```python
from build123d import *

# Parameters (mm, degrees)
SKETCH1_W           = 250
SKETCH1_H           = 176
BASE_FLANGE1_DEPTH  = 10
SKETCH6_W           = 50
SKETCH6_H           = 8
BOSS_EXTRUDE1_DEPTH = 10
SKETCH7_R           = 2
CUT_EXTRUDE1_DEPTH  = 158.927198417
SKETCH8_W           = 150
SKETCH8_H           = 76
CUT_EXTRUDE2_DEPTH  = 158.927198417
FILLET1_R           = 10


# Sheet-metal steps are written as plain solids
with BuildPart() as part:
    # Sketch1 → Base-Flange1 (new body)
    with BuildSketch(Plane(origin=(0, 0, 0), x_dir=(1, 0, 0), z_dir=(0, 1, 0))):
        Rectangle(SKETCH1_W, SKETCH1_H)
    extrude(amount=-BASE_FLANGE1_DEPTH)

    # Sketch6 → Boss-Extrude1 (add)
    with BuildSketch(Plane(origin=(0, 0, 0), x_dir=(1, 0, 0), z_dir=(0, 1, 0))):
        with Locations((0, 92)):
            Rectangle(SKETCH6_W, SKETCH6_H)
        with Locations((0, -92)):
            Rectangle(SKETCH6_W, SKETCH6_H)
    extrude(amount=-BOSS_EXTRUDE1_DEPTH)

    # Sketch7 → Cut-Extrude1 (cut, through all)
    with BuildSketch(Plane(origin=(0, 0, 0), x_dir=(1, 0, 0), z_dir=(0, 1, 0))):
        with Locations((25.707106781, 88.707106781)):
            Circle(SKETCH7_R)
        with Locations((-25.707106781, 88.707106781)):
            Circle(SKETCH7_R)
        with Locations((-25.707106781, -88.707106781)):
            Circle(SKETCH7_R)
        with Locations((25.707106781, -88.707106781)):
            Circle(SKETCH7_R)
    extrude(amount=-CUT_EXTRUDE1_DEPTH, mode=Mode.SUBTRACT)

    # Sketch8 → Cut-Extrude2 (cut, through all)
    with BuildSketch(Plane(origin=(0, 0, 0), x_dir=(1, 0, 0), z_dir=(0, 1, 0))):
        Rectangle(SKETCH8_W, SKETCH8_H)
    extrude(amount=-CUT_EXTRUDE2_DEPTH, mode=Mode.SUBTRACT)

    # Fillet1
    fillet1_edges = [part.edges().sort_by_distance(p)[0] for p in [
        (-75, -5, 38),
        (-75, -5, -38),
        (75, -5, -38),
        (75, -5, 38),
    ]]
    fillet(fillet1_edges, radius=FILLET1_R)


solid = part.part
```
Input: part model. Units: mm. Frame: model coordinates. A direction names the side the tool comes from. Give positions to 0.01 mm unless a question says otherwise; leave off trailing zeros. Order: outer loops, then holes, each group sorted by start corner. A loop starts at its lowest first (then second) coordinate and runs counter-clockwise, first axis right, second up. Notation, with made-up numbers: M 66,58 L 97,58 A22 ccw 97,89 Z; hole C 60,4.25 d9. An arc over 180 degrees is marked long. One line per question, with ' | ' between items.
1) Ray query, L1, parallel to X at y = -1.75, z = -10; L2, parallel to Z at x = -11, y = -9; L3, parallel to Z at x = 42, y = -6.5. Return the intervals inside material, ascending.
Filled in:
L1: x = -125 to -75, 75 to 125 | L2: z = -96 to -38, 38 to 96 | L3: z = -88 to -38, 38 to 88
2) Section D-D on x = 94.5. Output: boundary loops of the cut face in (y, z), and give its area (3 significant figures).
Filled in:
outline: M -10,-88 L 0,-88 L 0,88 L -10,88 Z | area: 1,760 mm2
3) Draft query along Z for faces 4 (the face through (76, -5, 88)), 5 (the face through (25, -5, -93)), 6 (the face through (71.99, -5.07, 35.15)). Return one class per face: pulls with the +Z half, pulls with the -Z half, needs draft (parallel to the pull), parting line crosses it, or undercut.
Filled in:
face 4: pulls with the +Z half | face 5: needs draft | face 6: undercut
4) Contact query for flat-ended pins moving along their axis: P1, Ø1.6, axis at y = -3.5, z = -93.5, coming from the +X side; P2, Ø6, axis at y = -4, z = 92.5, coming from the -X side; P3, Ø2, axis at x = 70.5, y = -2.5, coming from the +Z side. Output: stop coordinate, or through.
Filled in:
P1: stops at x = 25 | P2: stops at x = -25 | P3: stops at z = 88
5) Section B-B on x = -62. Output: boundary loops of the cut face in (y, z).
Filled in:
outline: M -10,-88 L 0,-88 L 0,-38 L -10,-38 Z; M -10,38 L 0,38 L 0,88 L -10,88 Z
6) Section A-A on z = -11. Output: boundary loops of the cut face in (x, y).
Filled in:
outline: M -125,-10 L -75,-10 L -75,0 L -125,0 Z; M 75,-10 L 125,-10 L 125,0 L 75,0 Z
7) Section C-C on y = -4. Output: boundary loops of the cut face in (x, z).
Filled in:
outline: M -125,-88 L -27.58,-88 A2 cw long -25,-90.58 L -25,-96 L 25,-96 L 25,-90.58 A2 cw long 27.58,-88 L 125,-88 L 125,88 L 27.58,88 A2 cw long 25,90.58 L 25,96 L -25,96 L -25,90.58 A2 cw long -27.58,88 L -125,88 Z; hole M -75,-28 A10 ccw -65,-38 L 65,-38 A10 ccw 75,-28 L 75,28 A10 ccw 65,38 L -65,38 A10 ccw -75,28 Z
8) Access query for faces 1 (the face through (25, -5, 93)), 2 (the face through (-77, -5, 88)), 3 (the face through (-71.99, -5.07, -35.15)). Directions: +Z, -Z, +X, -X, +Y, -Y. A direction counts if a zero-diameter tool reaches every point of the face in a straight line with its end or side. Return the directions, or none.
Filled in:
face 1: +Z, +X, +Y, -Y | face 2: +Z, -X, +Y, -Y | face 3: +Y, -Y
